from build123d import *

# Parameters (mm, degrees)
F1_DEPTH     = 76.2
F2_SIZE      = 25.4
F3_T1_DEPTH  = 325.0997163693
F3_T3_DEPTH  = 325.0997163693
F3_T5_DEPTH  = 247.368026375
F3_T7_DEPTH  = 325.557153853
F3_T9_DEPTH  = 263.50961712
F3_T11_DEPTH = 247.368026375
F3_T13_DEPTH = 247.368026375
F3_T15_DEPTH = 247.368026375
F3_T17_DEPTH = 247.368026375
F3_T19_DEPTH = 247.368026375
F3_T24_DEPTH = 324.0493372034
F3_T29_DEPTH = 324.0493372034
F3_T34_DEPTH = 247.368026375
F3_T39_DEPTH = 247.368026375


# Not quite as in the source:
# - a fillet or chamfer that OpenCascade refuses, or shapes differently, is made with other operations: its cross-section is extruded or revolved along the edge and cut away or added


with BuildPart() as f1:
    # F0 (on Front) → F1 (new body)
    with BuildSketch(Plane.XZ):
        Polygon((-22.9806532577, 64.0975162387), (-46.7637702823, 55.5351264775), (-60.4687564512, 34.2954342025), (-63.3636489511, 8.723853156), (-59.7226433456, -15.2280917391), (-25.1116699455, -37.9793605928), (0, -35.0888232076), (21.8782797456, -22.4281735718), (32.7606478844, 0.3868486179), (32.7606478844, 25.6643321522), (22.3381376327, 48.6930632045), (2.2968302766, 64.0975162387), align=None)
    extrude(amount=F1_DEPTH)

    # F2
    f2_edges = [f1.edges().sort_by_distance(p)[0] for p in [
        (-61.543146, -76.2, -3.252119),
        (-42.417157, -76.2, -26.603726),
        (-12.555835, -76.2, -36.534092),
        (10.93914, -76.2, -28.758498),
        (27.319464, -76.2, -11.020662),
        (32.760648, -76.2, 13.02559),
        (27.549393, -76.2, 37.178698),
        (12.317484, -76.2, 56.39529),
        (-10.341911, -76.2, 64.097516),
        (-34.872212, -76.2, 59.816321),
        (-53.616263, -76.2, 44.91528),
        (-61.916203, -76.2, 21.509644),
    ]]
    chamfer(f2_edges, length=F2_SIZE)

    # F3: chamfer of 43.18 on 12 edges, made by hand

    # F3_s2 → F3_t1 (cut)
    with BuildSketch(Plane.YZ.offset(-211.7576146723)):
        Polygon((-43.18, 64.0975162387), (0, 20.9175162387), (0, 64.0975162387), align=None)
    extrude(amount=F3_T1_DEPTH, mode=Mode.SUBTRACT)

    # F3_s4 → F3_t3 (cut)
    with BuildSketch(Plane(origin=(177.7014842233, 0, 63.9760283522), x_dir=(0, 1, 0), z_dir=(-0.9408815158, 0, -0.3387358457))):
        Polygon((0, -24.9125392558), (-43.18, -68.0925392558), (0, -68.0925392558), align=None)
    extrude(amount=F3_T3_DEPTH, mode=Mode.SUBTRACT)

    # F3_s6 → F3_t5 (cut)
    with BuildSketch(Plane(origin=(71.76035528, 0, 111.212652454), x_dir=(0, 1, 0), z_dir=(-0.5421815882, 0, -0.8402613435))):
        Polygon((0, -26.2239115206), (-43.18, -69.4039115206), (0, -69.4039115206), align=None)
    extrude(amount=F3_T5_DEPTH, mode=Mode.SUBTRACT)

    # F3_s8 → F3_t7 (cut)
    with BuildSketch(Plane(origin=(15.5595712054, 0, 137.4430436178), x_dir=(0, 1, 0), z_dir=(-0.1124888822, 0, -0.9936529834))):
        Polygon((0, -20.7628153082), (-43.18, -63.9428153082), (0, -63.9428153082), align=None)
    extrude(amount=F3_T7_DEPTH, mode=Mode.SUBTRACT)

    # F3_s10 → F3_t9 (cut)
    with BuildSketch(Plane(origin=(-127.5057052722, 0, 83.8149377508), x_dir=(0, 1, 0), z_dir=(0.8356288498, 0, -0.5492944796))):
        Polygon((0, -2.3503510843), (-43.18, -45.5303510843), (0, -45.5303510843), align=None)
    extrude(amount=F3_T9_DEPTH, mode=Mode.SUBTRACT)

    # F3_s12 → F3_t11 (cut)
    with BuildSketch(Plane(origin=(-139.4146792436, 0, -16.0476520785), x_dir=(0, 1, 0), z_dir=(0.9934402652, 0, 0.1143522606))):
        Polygon((0, 8.3213501676), (-43.18, -34.8586498324), (0, -34.8586498324), align=None)
    extrude(amount=F3_T11_DEPTH, mode=Mode.SUBTRACT)

    # F3_s14 → F3_t13 (cut)
    with BuildSketch(Plane(origin=(-111.323834941, 0, -64.4215215589), x_dir=(0, 1, 0), z_dir=(0.8655244386, 0, 0.500866695))):
        Polygon((0, 12.8097659916), (-43.18, -30.3702340084), (0, -30.3702340084), align=None)
    extrude(amount=F3_T13_DEPTH, mode=Mode.SUBTRACT)

    # F3_s16 → F3_t15 (cut)
    with BuildSketch(Plane(origin=(-52.4668465727, 0, -109.9974062184), x_dir=(0, 1, 0), z_dir=(0.4305162784, 0, 0.9025828128))):
        Polygon((0, 13.7773469096), (-43.18, -29.4026530904), (0, -29.4026530904), align=None)
    extrude(amount=F3_T15_DEPTH, mode=Mode.SUBTRACT)

    # F3_s18 → F3_t17 (cut)
    with BuildSketch(Plane.XY.offset(-110.6584228025)):
        Polygon((-10.4193521156, 0), (32.7606478844, -43.18), (32.7606478844, 0), align=None)
    extrude(amount=F3_T17_DEPTH, mode=Mode.SUBTRACT)

    # F3_s20 → F3_t19 (cut)
    with BuildSketch(Plane(origin=(41.7156753309, 0, -92.1715637275), x_dir=(0, 1, 0), z_dir=(-0.4123238865, 0, 0.9110373278))):
        Polygon((0, 2.7518097175), (-43.18, -40.4281902825), (0, -40.4281902825), align=None)
    extrude(amount=F3_T19_DEPTH, mode=Mode.SUBTRACT)


with BuildPart() as f3_tool22:
    # F3_s23 → F3_t24 (new body)
    with BuildSketch(Plane(origin=(-31.0979390453, 0, 204.5742860839), x_dir=(0, 1, 0), z_dir=(0.150286454, 0, -0.9886424944))):
        Polygon((0, -18.1529189981), (-43.18, -61.3329189981), (0, -61.3329189981), align=None)
    extrude(amount=F3_T24_DEPTH)

    split(bisect_by=Plane(origin=(-10.3155166871, 10.3814076541, 1.1677929431), x_dir=(-0.7093543397, -0.7048520559, 0), z_dir=(-0.7026187627, 0.7071067812, 0.0795416514)), keep=Keep.TOP)


with BuildPart() as f1_1:
    add(f1.part)

    # F3_t21: cut F3_tool22
    add(f3_tool22.part, mode=Mode.SUBTRACT)


with BuildPart() as f3_tool27:
    # F3_s28 → F3_t29 (new body)
    with BuildSketch(Plane(origin=(-31.0979390453, 0, 204.5742860839), x_dir=(0, 1, 0), z_dir=(0.150286454, 0, -0.9886424944))):
        Polygon((0, -18.1529189981), (-43.18, -61.3329189981), (0, -61.3329189981), align=None)
    extrude(amount=F3_T29_DEPTH)

    split(bisect_by=Plane(origin=(-0.6455174379, 1.1751755422, -0.9820105866), x_dir=(-0.876476897, -0.481443921, 0), z_dir=(-0.3884098514, 0.7071067812, -0.5908788263)), keep=Keep.TOP)


with BuildPart() as f1_2:
    add(f1_1.part)

    # F3_t26: cut F3_tool27
    add(f3_tool27.part, mode=Mode.SUBTRACT)


with BuildPart() as f3_tool32:
    # F3_s33 → F3_t34 (new body)
    with BuildSketch(Plane(origin=(78.5572793932, 0, -60.3818852432), x_dir=(0, 1, 0), z_dir=(-0.7928521575, 0, 0.609414027))):
        Polygon((-43.18, -52.2195746281), (0, -9.0395746281), (0, -52.2195746281), align=None)
    extrude(amount=F3_T34_DEPTH)

    split(bisect_by=Plane(origin=(-1.2535006858, -1.3759048587, -0.5673184388), x_dir=(-0.7392234901, 0.6734601931, 0), z_dir=(0.6442006724, 0.7071067812, 0.2915570162)), keep=Keep.TOP)


with BuildPart() as f1_3:
    add(f1_2.part)

    # F3_t31: cut F3_tool32
    add(f3_tool32.part, mode=Mode.SUBTRACT)


with BuildPart() as f3_tool37:
    # F3_s38 → F3_t39 (new body)
    with BuildSketch(Plane(origin=(78.5572793932, 0, -60.3818852432), x_dir=(0, 1, 0), z_dir=(-0.7928521575, 0, 0.609414027))):
        Polygon((-43.18, -52.2195746281), (0, -9.0395746281), (0, -52.2195746281), align=None)
    extrude(amount=F3_T39_DEPTH)

    split(bisect_by=Plane(origin=(0, 10.4587581193, 10.4587581193), x_dir=(1, 0, 0), z_dir=(0, 0.7071067812, 0.7071067812)), keep=Keep.TOP)


with BuildPart() as f1_4:
    add(f1_3.part)

    # F3_t36: cut F3_tool37
    add(f3_tool37.part, mode=Mode.SUBTRACT)


solid = f1_4.part
CAD build for the part. Positions are in the model's coordinates, mm. Coordinates: 2 decimals unless noted, no trailing zeros. Write each loop counter-clockwise with the first axis right and the second up, starting at its lowest first coordinate (ties: lowest second). Pieces come first, ordered by that corner, then holes. Notation, with made-up numbers: M 24,-33.75 L 32,-33.75 A9 cw 32,-25.75 Z; hole C -6.5,76 d5. An arc over 180 degrees is marked long. Answer as a JSON object with one key per item and string values. Group by question number.
1) Saw through at C-C (x = 5). Write the cut outline in (y, z).
2) Saw through at A-A (y = -58.5). Write the cut outline in (x, z), plus the area to 3 significant figures.
3) Saw through at D-D (y = -34). Write the cut outline in (x, z), plus the area to 3 significant figures.
4) Pin check, flat tips, straight feed: pin 1 Ø6 at (x, y) = (-53.5, -37) entering from +Z; pin 2 Ø8 at (x, y) = (-29.5, -50) entering from -Z; pin 3 Ø1.5 at (x, y) = (-36.5, -21.5) entering from +Z. Stop position of each tip, or through.
5) Wall check: line 1 (X direction, y = -42.5, z = 6); line 2 (Y direction, x = -4.5, z = 46.5); line 3 (Z direction, x = -48, y = -60). Give the ranges that are in metal, low to high. Write a range as from..to.
6) Saw through at B-B (z = 29.5). Write the cut outline in (x, y), plus the area to 3 significant figures.
Values follow:
{
 "1": {"outline": "M -76.2,1.19 L -72.74,-6.84 L -50.8,-32.2 L -43.18,-32.2 L -21.24,-6.84 L -15.42,6.67 L -15.42,19.67 L -27.11,48.03 L -41.1,62.02 L -50.8,62.02 L -72.26,34.95 L -76.2,25.4 Z"},
 "2": {"outline": "M -55.6,8.87 L -52.63,-10.68 L -23.22,-30.01 L -2.47,-27.62 L 15.96,-16.96 L 25.06,2.13 L 25.06,24 L 16.12,43.76 L -0.32,56.4 L -21.64,56.4 L -41.71,49.17 L -53.02,31.64 Z", "area": "5,570 mm2"},
 "3": {"outline": "M -55.88,-6.77 L -22.85,-28.48 L -2.95,-26.19 L 14.82,-15.91 L 23.58,2.46 L 23.58,23.68 L 9.44,54.92 L -21.38,54.92 L -40.73,47.95 L -51.59,31.13 Z", "area": "5,280 mm2"},
 "4": {"pin 1": "stops at z = 40.92", "pin 2": "stops at z = -37.72", "pin 3": "stops at z = 33.26"},
 "5": {"line 1": "x = -62.95..32.08", "line 2": "y = -68.4..-25.58", "line 3": "z = -11.92..36.65"},
 "6": {"outline": "M -61.01,-50.8 L -47.04,-64.69 L -33.33,-76.2 L 3.14,-76.2 L 31.02,-50.8 L 31.02,-43.18 L -6.95,-8.58 L -16.94,-8.58 L -26.07,-11.67 L -47.04,-29.29 L -61.01,-43.18 Z", "area": "4,230 mm2"}
}
